Geometry check sheet. Reference: the model listing, model coordinates, mm. Coordinates: 2 decimals unless noted, no trailing zeros. Write each loop counter-clockwise with the first axis right and the second up, starting at its lowest first coordinate (ties: lowest second). Pieces come first, ordered by that corner, then holes. Notation, with made-up numbers: (74.25, 10) -> (106.25, 10) arc R7 cw to (106.25, 15) -> close; hole circle Ø3 at (-31, 18). An arc over 180 degrees is marked (long way). One line per question, with ' | ' between items.
from build123d import *

# Parameters (mm, degrees)
SKETCH2_R           = 1.5
SKETCH2_W           = 5
SKETCH2_H           = 120
BOSS_EXTRUDE1_DEPTH = 5
SKETCH3_R           = 1
SKETCH3_W           = 5
SKETCH3_H           = 180
CUT_EXTRUDE1_DEPTH  = 5
FILLET1_R           = 10
SKETCH4_W           = 10
SKETCH4_H           = 10
CUT_EXTRUDE2_DEPTH  = 10


with BuildPart() as part:
    # Sketch2 → Boss-Extrude1 (new body)
    with BuildSketch(Plane(origin=(0, 0, 0), x_dir=(1, 0, 0), z_dir=(0, 1, 0))):
        Polygon((0, 375), (0, 0), (0, -230), (10, -230), (15, -230), (117.5, -230), (117.5, 475), (127.5, 475), (127.5, -230), (230, -230), (235, -230), (245, -230), (245, -10), (245, 355), (245.3, 385), (245.3, 590), (245, 590), (0, 590), (-0.3, 590), (-0.3, 405), align=None)
        with Locations((66.25, -225)):
            Circle(SKETCH2_R, mode=Mode.SUBTRACT)
        with Locations((12.5, 140)):
            Rectangle(SKETCH2_W, SKETCH2_H, mode=Mode.SUBTRACT)
        with Locations((178.75, -225)):
            Circle(SKETCH2_R, mode=Mode.SUBTRACT)
        with Locations((232.5, 140)):
            Rectangle(SKETCH2_W, SKETCH2_H, mode=Mode.SUBTRACT)
        with Locations((12.5, 320)):
            Rectangle(SKETCH2_W, SKETCH2_H, mode=Mode.SUBTRACT)
        with Locations((12.5, 500)):
            Rectangle(SKETCH2_W, SKETCH2_H, mode=Mode.SUBTRACT)
        with Locations((66.25, 585)):
            Circle(SKETCH2_R, mode=Mode.SUBTRACT)
        with Locations((232.5, 320)):
            Rectangle(SKETCH2_W, SKETCH2_H, mode=Mode.SUBTRACT)
        with Locations((178.75, 585)):
            Circle(SKETCH2_R, mode=Mode.SUBTRACT)
        with Locations((232.5, 500)):
            Rectangle(SKETCH2_W, SKETCH2_H, mode=Mode.SUBTRACT)
    extrude(amount=BOSS_EXTRUDE1_DEPTH)

    # Sketch3 → Cut-Extrude1 (cut)
    with BuildSketch(Plane(origin=(0, 5, 0), x_dir=(1, 0, 0), z_dir=(0, 1, 0))):
        with Locations((17, 420)):
            Circle(SKETCH3_R)
        with Locations((17, 430)):
            Circle(SKETCH3_R)
        with Locations((102.5, 130)):
            Rectangle(SKETCH3_W, SKETCH3_H)
    cut_extrude1 = extrude(amount=-CUT_EXTRUDE1_DEPTH, mode=Mode.SUBTRACT)

    # Mirror1: Cut-Extrude1 across plane
    add(cut_extrude1.mirror(Plane.ZY.offset(-122.5)), mode=Mode.SUBTRACT)

    # Fillet1
    fillet1_edges = [part.edges().sort_by_distance(p)[0] for p in [
        (245, 2.5, 230),
        (0, 2.5, 230),
        (-0.3, 2.5, -590),
        (245.3, 2.5, -590),
    ]]
    fillet(fillet1_edges, radius=FILLET1_R)

    # Sketch4 → Cut-Extrude2 (cut)
    with BuildSketch(Plane(origin=(0, 5, 0), x_dir=(1, 0, 0), z_dir=(0, 1, 0))):
        with Locations((15, -225)):
            Rectangle(SKETCH4_W, SKETCH4_H)
        with Locations((230, -225)):
            Rectangle(SKETCH4_W, SKETCH4_H)
        with Locations((14.7, 585)):
            Rectangle(SKETCH4_W, SKETCH4_H)
        with Locations((230.3, 585)):
            Rectangle(SKETCH4_W, SKETCH4_H)
        with Locations((122.5, 585)):
            Rectangle(SKETCH4_W, SKETCH4_H)
    extrude(amount=-CUT_EXTRUDE2_DEPTH, mode=Mode.SUBTRACT)


solid = part.part
1. Cross-section at B-B on z = -131.5. Record the boundary of the cut face in (x, y).
Worked answers:
outline: (0, 0) -> (10, 0) -> (10, 5) -> (0, 5) -> close; (15, 0) -> (100, 0) -> (100, 5) -> (15, 5) -> close; (105, 0) -> (117.5, 0) -> (117.5, 5) -> (105, 5) -> close; (127.5, 0) -> (140, 0) -> (140, 5) -> (127.5, 5) -> close; (145, 0) -> (230, 0) -> (230, 5) -> (145, 5) -> close; (235, 0) -> (245, 0) -> (245, 5) -> (235, 5) -> close
2. Go/stop test with flat-tipped pins: P1, Ø1.5, axis at x = 13, y = 1.5, coming from the -Z side; P2, Ø2.5, axis at x = 231.5, y = 2.5, coming from the +Z side; P3, Ø2.5, axis at x = 228, z = -430, coming from the -Y side; P4, Ø2.5, axis at y = 1.5, z = -316, coming from the -X side. Record where each tip stops, or that it passes through.
Worked answers:
P1: z = -580 | P2: z = 220 | P3: y = 0 | P4: x = 0
3. Material ranges on line 1 (X direction, y = 3.25, z = -540); line 2 (X direction, y = 0.6, z = -175); line 3 (Z direction, x = 17, y = 3.3), recorded low to high. Write a range as from..to.
Worked answers:
line 1: -0.3..10, 15..230, 235..245.3 | line 2: 0..10, 15..100, 105..117.5, 127.5..140, 145..230, 235..245 | line 3: -580..-431, -429..-421, -419..220
4. Cross-section at C-C on y = 1.5. Give the number of separate pieces and of enclosed holes in the cut face, and give its area (3 significant figures).
Worked answers:
separate pieces: 1 | enclosed holes: 16 | area: 188,000 mm²
5. Cross-section at A-A on z = -339. Record the boundary of the cut face in (x, y).
Worked answers:
outline: (0, 0) -> (10, 0) -> (10, 5) -> (0, 5) -> close; (15, 0) -> (117.5, 0) -> (117.5, 5) -> (15, 5) -> close; (127.5, 0) -> (230, 0) -> (230, 5) -> (127.5, 5) -> close; (235, 0) -> (245, 0) -> (245, 5) -> (235, 5) -> close
